The model under review builds one solid part; all positions refer to its coordinate system, in mm. Face numbers are marked on the shaded views. A direction names the side the tool comes from. Round coordinates to 2 decimals unless told otherwise and drop trailing zeros. Loops run counter-clockwise (first coordinate to the right, second up) from the corner with the lowest first, then second, coordinate; pieces in that order, holes last. Notation, with made-up numbers: M 86.25,-39.75 L 111.25,-39.75 A34 cw 111.25,-1.75 Z; hole C 14.25,36 d2. An arc over 180 degrees is marked long. Use a Markdown table: item, result. Add a question column.
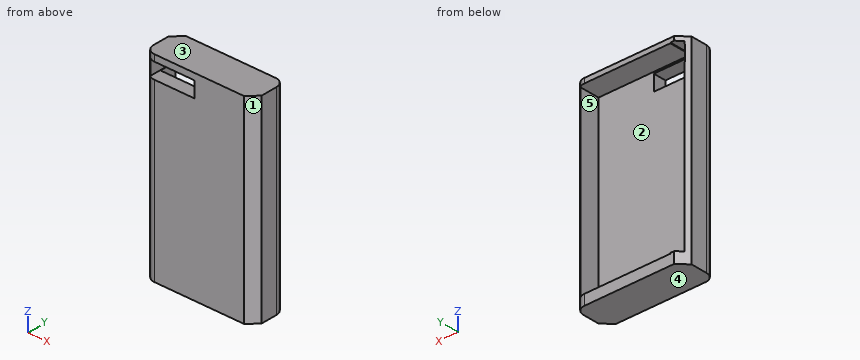
```python
from build123d import *

# Parameters (mm, degrees)
F0_W         = 59.69
F0_H         = 109.22
F1_DEPTH     = 19.304
F2_W         = 50.8
F2_H         = 100.838
F3_DEPTH     = 12.192
F4_W         = 5.1237940788
F4_H         = 100.838
F5_DEPTH     = 12.192
F6_W         = 25.4
F6_H         = 8.6614
F7_DEPTH     = 45.974
F8_T1_DEPTH  = 134.62
F9_SIZE      = 5.08
F10_T1_DEPTH = 134.62
F11_T1_DEPTH = 135.3482991577


# Not quite as in the source:
# - a fillet or chamfer that OpenCascade refuses, or shapes differently, is made with other operations: its cross-section is extruded or revolved along the edge and cut away or added


with BuildPart() as f1:
    # F0 (on Front) → F1 (new body)
    with BuildSketch(Plane.XZ):
        with Locations((1.3794824481, 0)):
            Rectangle(F0_W, F0_H)
    extrude(amount=F1_DEPTH)

    # F2 (on Front) → F3 (cut)
    with BuildSketch(Plane.XZ):
        with Locations((3.9194825381, 1.5458958449)):
            Rectangle(F2_W, F2_H)
    extrude(amount=F3_DEPTH, mode=Mode.SUBTRACT)

    # F4 (on Front) → F5 (cut)
    with BuildSketch(Plane.XZ):
        with Locations((-23.8453447819, 1.9400352838)):
            Rectangle(F4_W, F4_H)
    extrude(amount=F5_DEPTH, mode=Mode.SUBTRACT)

    # F6 (on Front) → F7 (cut)
    with BuildSketch(Plane.XZ):
        with Locations((-13.9043106094, 46.7005276281)):
            Rectangle(F6_W, F6_H)
    extrude(amount=F7_DEPTH, mode=Mode.SUBTRACT)

    # F8: fillet of radius 5.08 on 1 edges, made by hand

    # F8_s2 → F8_t1 (cut)
    with BuildSketch(Plane.XY.offset(-67.31)):
        with BuildLine():
            ThreePointArc((-28.4655175519, -14.224), (-26.9776200003, -17.8161024484), (-23.3855175519, -19.304))
            Line((-23.3855175519, -19.304), (-28.4655175519, -19.304))
            Line((-28.4655175519, -19.304), (-28.4655175519, -14.224))
        make_face()
    extrude(amount=F8_T1_DEPTH, mode=Mode.SUBTRACT)

    # F9
    f9_edges = [f1.edges().sort_by_distance(p)[0] for p in [
        (31.224482, -19.304, 0),
    ]]
    chamfer(f9_edges, length=F9_SIZE)

    # F10: fillet of radius 5.08 on 1 edges, made by hand

    # F10_s2 → F10_t1 (cut)
    with BuildSketch(Plane.XY.offset(-67.31)):
        with BuildLine():
            ThreePointArc((31.2244824481, -5.08), (29.7365848965, -1.4878975516), (26.1444824481, 0))
            Line((26.1444824481, 0), (31.2244824481, 0))
            Line((31.2244824481, 0), (31.2244824481, -5.08))
        make_face()
    extrude(amount=F10_T1_DEPTH, mode=Mode.SUBTRACT)

    # F11: chamfer of 5.08 on 1 edges, made by hand

    # F11_s2 → F11_t1 (cut)
    with BuildSketch(Plane.XY.offset(-67.6741495789)):
        Polygon((-28.4655175519, -5.08), (-23.3855175519, 0), (-28.4655175519, 0), align=None)
    extrude(amount=F11_T1_DEPTH, mode=Mode.SUBTRACT)


solid = f1.part
```
(1) Consider section B-B, the plane x = -17.5. Give the boundary of the cut face in (y, z).
(2) Draft analysis for pull direction X (two halves, no side actions). For the marked faces 1, 2 and 3, state which applies: released by +X, released by -X, zero draft, split by the parting line, or undercut.
(3) Consider section C-C, the plane z = 48. Give the boundary of the cut face in (x, y), then the cut area to 3 significant figures.
(4) Consider section A-A, the plane y = -8.5. Give the boundary of the cut face in (x, z).
(5) To check wall thickness, follow probe 1 along X at (y, z) = (-6.75, -6.5); probe 2 along Z at (x, y) = (-12, -10.5); probe 3 along Z at (x, y) = (-12, -14). State the ranges of each line that lie inside material, in increasing order.
(6) For the marked faces 4 and 5, list the 3-axis set-ups (+Z, -Z, +X, -X, +Y, -Y) from which the entire face can be reached by the end or side of a thin tool; tool diameter is ignored.
(7) Consider section D-D, the plane z = -16.5. Give the boundary of the cut face in (x, y).
(8) Insertion check: pin 1 Ø1.5 at (x, z) = (7.5, -4.5) entering from +Y; pin 2 Ø5.5 at (y, z) = (-17.5, 44.5) entering from -X. Each pin has a flat end and moves straight along its axis. Give the tip position at first contact, or say it passes through.
Found:
| question | item | result |
|---|---|---|
| 1 | outline | M -19.3,-54.61 L 0,-54.61 L 0,-48.87 L -12.19,-48.87 L -12.19,42.37 L -19.3,42.37 Z; M -19.3,51.03 L -12.19,51.03 L -12.19,51.96 L 0,51.96 L 0,54.61 L -19.3,54.61 Z |
| 2 | face 1 | released by +X |
| 2 | face 2 | undercut |
| 2 | face 3 | zero draft |
| 3 | outline | M -28.47,-14.22 A5.08 ccw -26.6,-18.15 L -26.6,-3.22 L -28.47,-5.08 Z; M -1.2,-19.3 L 26.14,-19.3 L 31.22,-14.22 L 31.22,-5.08 A5.08 ccw 29.32,-1.11 L 29.32,-12.19 L -1.2,-12.19 Z |
| 3 | area | 260 mm^2 |
| 4 | outline | M -28.47,-54.61 L 31.22,-54.61 L 31.22,54.61 L -28.47,54.61 Z; hole M -26.6,42.37 L -26.41,42.37 L -26.41,-48.48 L -21.48,-48.48 L -21.48,-48.87 L 29.32,-48.87 L 29.32,51.96 L -21.28,51.96 L -21.28,52.36 L -26.41,52.36 L -26.41,51.03 L -26.6,51.03 Z |
| 5 | probe 1 | x = -28.47 to -26.41, 29.32 to 31.22 |
| 5 | probe 2 | z = -54.61 to -48.87, 51.96 to 54.61 |
| 5 | probe 3 | z = -54.61 to 42.37, 51.03 to 54.61 |
| 6 | face 4 | -Z, +X, -X, +Y, -Y |
| 6 | face 5 | +Y |
| 7 | outline | M -28.47,-14.22 A5.08 ccw -23.39,-19.3 L 26.14,-19.3 L 31.22,-14.22 L 31.22,-5.08 A5.08 ccw 29.32,-1.11 L 29.32,-12.19 L -26.41,-12.19 L -26.41,-3.02 L -28.47,-5.08 Z |
| 8 | pin 1 | stops at y = -12.19 |
| 8 | pin 2 | stops at x = -28.44 |
